For this review, take the finished solid that the model builds, in its own axes (mm). A direction names the side the tool comes from. Coordinates: 2 decimals unless noted, no trailing zeros. Write each loop counter-clockwise with the first axis right and the second up, starting at its lowest first coordinate (ties: lowest second). Pieces come first, ordered by that corner, then holes. Notation, with made-up numbers: (4, -35.5) - (34, -35.5) arc R17 cw to (34, -21.5) - close; hole circle Ø2 at (65.25, -19). An arc over 180 degrees is marked (long way). Use one line per item in the form item = value. Start each with the question number.
1) Mouldability with a two-part tool opening along Y and no side actions: class faces 1 (the flat face through (179.768, -47, -276)), 2 (the flat face through (-6, 647.7, 6)), 3 (the flat face through (-253, 45, 217.891)) as pulls with the +Y half, pulls with the -Y half, needs draft (parallel to the pull), parting line crosses it, or undercut.
2) We need section A-A (y = -59). Give the boundary of the cut face in (x, z) (1 decimal).
3) For L1, parallel to Z at x = 0, y = 46; L2, parallel to Y at x = -145, z = 222; L3, parallel to Z at x = -149.5, y = -124.5, list the stretches that pass through material, from the lowest coordinate up. Write a range as from..to.
4) We need section C-C (z = 0). Give the boundary of the cut face in (x, y) (1 decimal), plus the area to 3 significant figures.
5) Insertion check: P1, Ø24, axis at y = -194, z = -283, coming from the +X side; P2, Ø1, axis at x = -46, z = 238.5, coming from the -Y side; P3, Ø1.5, axis at y = -440.5, z = 241.5, coming from the -X side. Each pin has a flat end and moves straight along its axis. Give the tip position at first contact, or say it passes through.
6) We need section B-B (x = 0). Give the boundary of the cut face in (y, z).
7) Tool access review of faces 4 (the flat face through (-179.779, -47, -276)), 5 (the flat face through (115, -647.7, 293)), 6 (the flat face through (-320, 219.075, 18)): name each direction out of +Z, -Z, +X, -X, +Y, -Y from which nothing blocks a thin tool from reaching the whole face with its end or side.
8) We need section D-D (y = -513.5). Give the boundary of the cut face in (x, z) (1 decimal).
```python
from build123d import *

# Parameters (mm, degrees)
F0_R     = 360.3625
F1_DEPTH = 647.7
F3_DEPTH = 1219.2
F5_W     = 342.9
F5_H     = 393.7
F6_DEPTH = 279.4
F7_R     = 393.7
F7_R_2   = 360.3625
F8_DEPTH = 647.7


# Not quite as in the source:
# - a feature names something its author has since deleted; it is built from what else it names


with BuildPart() as f1:
    # F0 (on Front) → F1 (new body, symmetric)
    with BuildSketch(Plane.XZ):
        Circle(F0_R)
    extrude(amount=F1_DEPTH, both=True)

    # F2 (on face) → F3 (cut)
    with BuildSketch(Plane.XZ.offset(647.7)):
        with BuildLine():
            ThreePointArc((-76.2, -300.0375), (-130.2228778271, -280.8397113954), (-179.7789835799, -252.0088460138))
            Line((-179.7789835799, -252.0088460138), (-179.7789835799, -300.0375))
            Line((-179.7789835799, -300.0375), (-76.2, -300.0375))
        make_face()
        with BuildLine():
            ThreePointArc((179.7685, -252.016324499), (275.2076740277, -141.7380596823), (309.5625, 0))
            ThreePointArc((309.5625, 0), (-141.7323354104, 275.2106220794), (-179.7789835799, -252.0088460138))
            ThreePointArc((-179.7789835799, -252.0088460138), (-130.2228778271, -280.8397113954), (-76.2, -300.0375))
            Line((-76.2, -300.0375), (76.2, -300.0375))
            ThreePointArc((76.2, -300.0375), (130.217036413, -280.8424199334), (179.7685, -252.016324499))
        make_face()
        with BuildLine():
            Line((179.7685, -300.0375), (179.7685, -252.016324499))
            ThreePointArc((179.7685, -252.016324499), (130.217036413, -280.8424199334), (76.2, -300.0375))
            Line((76.2, -300.0375), (179.7685, -300.0375))
        make_face()
    extrude(amount=-F3_DEPTH, mode=Mode.SUBTRACT)

    # F5 (on offset) → F6 (cut)
    with BuildSketch(Plane.YZ.offset(-203.2)):
        with Locations((47.625, 21.0411539862)):
            Rectangle(F5_W, F5_H)
    extrude(amount=-F6_DEPTH, mode=Mode.SUBTRACT)

    # F7 (on Front) → F8 (join, symmetric)
    with BuildSketch(Plane.XZ):
        Circle(F7_R)
        Circle(F7_R_2, mode=Mode.SUBTRACT)
    extrude(amount=F8_DEPTH, both=True)


solid = f1.part
```
Determined:
q1.face_1 = needs draft
q1.face_2 = pulls with the +Y half
q1.face_3 = undercut
q2.outline = circle Ø787.4 at (0, 0); hole (-314.6, -175.8) - (-254.8, -175.8) arc R309.6 ccw to (-179.8, -252) - (-179.8, -300) - (179.8, -300) - (179.8, -252) arc R309.6 ccw (long way) to (-219.9, 217.9) - (-287, 217.9) arc R360.4 ccw to start
q3.L1 = -393.7..-300.04, 309.56..393.7
q3.L2 = 571.5..647.7
q3.L3 = -364.21..-300.04, 271.07..364.21
q4.outline = (-393.7, -647.7) - (-309.6, -647.7) - (-309.6, -123.8) - (-360.4, -123.8) - (-360.4, 219.1) - (-309.6, 219.1) - (-309.6, 571.5) - (309.6, 571.5) - (309.6, -647.7) - (393.7, -647.7) - (393.7, 647.7) - (-393.7, 647.7) - close
q4.area = 248,000 mm²
q5.P1 = 285.58
q5.P2 = 571.5
q5.P3 = -311.51
q6.outline = (-647.7, -393.7) - (647.7, -393.7) - (647.7, 393.7) - (-647.7, 393.7) - (-647.7, 309.56) - (571.5, 309.56) - (571.5, -300.04) - (-647.7, -300.04) - close
q7.face_4 = -Y
q7.face_5 = +Z, -Z, +X, -X, -Y
q7.face_6 = none
q8.outline = circle Ø787.4 at (0, 0); hole (-179.8, -300) - (179.8, -300) - (179.8, -252) arc R309.6 ccw (long way) to (-179.8, -252) - close
